Autodesk Inventor part; units mm, degrees
ref_plane "Work Plane1" through (-3.175, -19.05, 12.7) normal (-1, 0, 0) x (0, 0, 1)
ref_plane "YZ Plane" through (0, 0, 0) normal (1, 0, 0) x (0, 1, 0)
ref_plane "XZ Plane" through (0, 0, 0) normal (0, 1, 0) x (-1, 0, 0)
sketch "Sketch1" plane through (0, 0, 0) normal (0, 0, 1) x (1, 0, 0)
  circle A0 centre (0, 0) radius 9.525 construction
  circle A1 centre (0, 0) radius 1.9812
  line L0 (-9.525, 19.05) -> (-9.525, -19.05)
  line L1 (-9.525, 19.05) -> (-3.175, 19.05)
  line L2 (-3.175, 19.05) -> (7.4009, 5.996)
  line L3 (-9.525, -19.05) -> (-3.175, -19.05)
  line L4 (-3.175, -19.05) -> (7.4009, -5.996)
  arc A2 (7.4009, -5.996) -> (7.4009, 5.996) centre (0, 0) ccw
  point P0 (-9.525, 0)
  dimension "d0" = 19.05
  dimension "d1" = 3.9624
  dimension "d3" = 38.1
  dimension "d17" = 6.35
  dimension "d26" = 9.525
extrude "Extrusion1" add sketch "Sketch1" along normal mid plane 25.4
sketch "Sketch2" plane through (-9.525, -19.05, 12.7) normal (-1, 0, 0) x (0, 0, 1)
  circle A0 centre (-12.7, 19.05) radius 2.4892 construction
  line L0 (-25.4, 0) -> (-25.4, 38.1)
  circle A1 centre (-12.7, 31.75) radius 2.4892
  circle A2 centre (-12.7, 6.35) radius 2.4892
  circle A3 centre (-12.7, 19.05) radius 2.4892 construction
  dimension "d6" = 4.9784
  dimension "d9" = 12.7
  dimension "d12" = 12.7
extrude "Extrusion2" cut sketch "Sketch2" against normal through all
ref_plane "Work Plane1" through (-3.175, -19.05, 12.7) normal (-1, 0, 0) x (0, 0, 1)
sketch "Sketch3" plane through (-3.175, -19.05, 12.7) normal (-1, 0, 0) x (0, 0, 1)
  circle A0 centre (-12.7, 31.75) radius 2.4892
  circle A1 centre (-12.7, 6.35) radius 2.4892
  circle A2 centre (-12.7, 31.75) radius 5.2705
  circle A3 centre (-12.7, 6.35) radius 5.2705
  point P0 (-12.7, 19.05)
  dimension "d18" = 10.541
  dimension "d19" = 10.541
extrude "Extrusion3" cut sketch "Sketch3" against normal through all
thread "Thread1"
fillet "Fillet1" radius 6.35 4 edges at (-6.35, 19.05, 12.7) (-6.35, 19.05, -12.7) (-6.35, -19.05, 12.7) (-6.35, -19.05, -12.7)
sketch "Sketch5" plane through (0, 0, -12.7) normal (0, 0, -1) x (-1, 0, 0)
  circle A0 centre (0, 0) radius 1.9812
extrude "Extrusion5" [suppressed]
equation "\"d19\" = d18"
properties part number "F4C9-200-002 Side Bearing Block" material "Aluminum 6061"
The model under review builds one solid part; all positions refer to its coordinate system, in mm. A direction names the side the tool comes from. Coordinates: 2 decimals unless noted, no trailing zeros. Loops run counter-clockwise (first coordinate to the right, second up) from the corner with the lowest first, then second, coordinate; pieces in that order, holes last. Notation, with made-up numbers: (4, 49.5) -> (16, 49.5) arc R22 cw to (16, 82.5) -> close; hole circle Ø4 at (33, -20). An arc over 180 degrees is marked (long way). Use a Markdown table: item, result. Add a question column.
1. Add section B-B on y = 0. Write out the cut boundary in (x, z) (3 decimals), plus the area to 3 significant figures.
2. Draft analysis for pull direction Y (two halves, no side actions). For faces 1 (the face through (-6.39, -10.6, 1.34)), 2 (the face through (-9.525, 0, 0)), 3 (the face through (2.04, 12.61, -5.82)), state which applies: pulls with the +Y half, pulls with the -Y half, needs draft (parallel to the pull), parting line crosses it, or undercut.
3. Add section A-A on z = 0. Give the number of separate pieces and of enclosed holes in the cut face, plus the area to 3 significant figures.
4. Machinability: for faces 4 (the face through (-3.175, -13.8, -2.4)), 5 (the face through (-6, 19.05, 0)), which of the approach directions +Z, -Z, +X, -X, +Y, -Y give a long, thin tool a straight path to every point of the face, cutting with its end or side? Answer none if there is none.
5. Add section D-D on z = -4. Write out the cut boundary in (x, y) (3 decimals), plus the area to 3 significant figures.
6. Clearance check with flat-ended pins moving along their axes: pin 1 Ø6 at (x, z) = (2, -5.5) entering from +Y; pin 2 Ø1.5 at (x, z) = (-1, 1.5) entering from +Y; pin 3 Ø5 at (x, z) = (6, -10) entering from -Y; pin 4 Ø4.5 at (y, z) = (12.7, 0) entering from -X. State where each tip first meets the part, or that it passes through.
7. Add section C-C on x = -3.75. Write out the cut boundary in (y, z).
8. To check wall thickness, follow line 1 (Y direction, x = -4.5, z = 0); line 2 (Z direction, x = 0, y = 12.7); line 3 (X direction, y = -6, z = -1.25) (3 decimals). State the ranges of each line that lie inside material, in increasing order.
Returned:
| question | item | result |
|---|---|---|
| 1 | outline | (-9.525, -12.7) -> (-1.981, -12.7) -> (-1.981, 12.7) -> (-9.525, 12.7) -> close; (1.981, -12.7) -> (9.525, -12.7) -> (9.525, 12.7) -> (1.981, 12.7) -> close |
| 1 | area | 383 mm² |
| 2 | face 1 | undercut |
| 2 | face 2 | needs draft |
| 2 | face 3 | pulls with the +Y half |
| 3 | separate pieces | 3 |
| 3 | enclosed holes | 1 |
| 3 | area | 340 mm² |
| 4 | face 4 | +X |
| 4 | face 5 | +Z, -Z, +X, -X, +Y |
| 5 | outline | (-9.525, -19.05) -> (-3.175, -19.05) -> (-0.811, -16.132) -> (-3.175, -16.132) -> (-3.175, -9.268) -> (4.75, -9.268) -> (7.401, -5.996) arc R9.525 ccw to (7.401, 5.996) -> (4.75, 9.268) -> (-3.175, 9.268) -> (-3.175, 16.132) -> (-0.811, 16.132) -> (-3.175, 19.05) -> (-9.525, 19.05) -> close; hole circle Ø3.962 at (0, 0) |
| 5 | area | 441 mm² |
| 6 | pin 1 | stops at y = 16.37 |
| 6 | pin 2 | stops at y = 7.93 |
| 6 | pin 3 | stops at y = -10.81 |
| 6 | pin 4 | passes through |
| 7 | outline | (-19.05, -6.35) arc R6.35 ccw to (-12.7, -12.7) -> (12.7, -12.7) arc R6.35 ccw to (19.05, -6.35) -> (19.05, 6.35) arc R6.35 ccw to (12.7, 12.7) -> (-12.7, 12.7) arc R6.35 ccw to (-19.05, 6.35) -> close; hole circle Ø4.98 at (-12.7, 0); hole circle Ø4.98 at (12.7, 0) |
| 8 | line 1 | y = -19.05 to -15.19, -10.21 to 10.21, 15.19 to 19.05 |
| 8 | line 2 | z = -12.7 to -5.27, 5.27 to 12.7 |
| 8 | line 3 | x = -9.525 to 7.398 |
